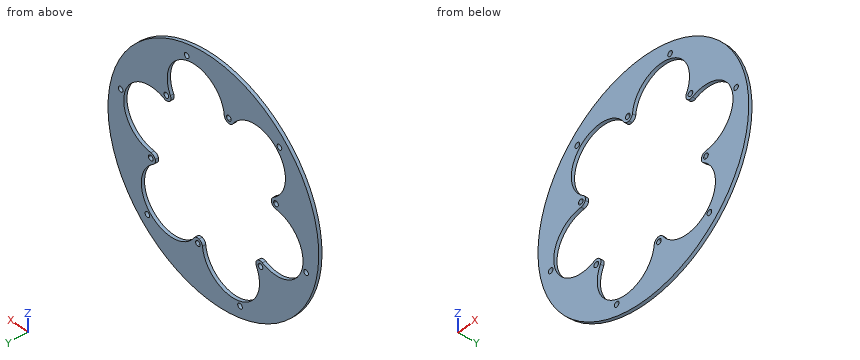
from build123d import *

# Parameters (mm, degrees)
SKETCH1_R           = 90.5
SKETCH1_R_2         = 2
BOSS_EXTRUDE1_DEPTH = 2.5


with BuildPart() as part:
    # Sketch1 → Boss-Extrude1 (new body)
    with BuildSketch(Plane(origin=(0, 0, 0), x_dir=(1, 0, 0), z_dir=(0, 1, 0))):
        with Locations(Location((0, 0, 0), (0, 0, 270))):
            Circle(SKETCH1_R)
        with Locations(Location((-56.728619257, -59.210334885, 0), (0, 0, 270))):
            Circle(SKETCH1_R_2, mode=Mode.SUBTRACT)
        with BuildLine():
            ThreePointArc((-13.809474495, -56.333511054), (-15.279862915, -53.913851845), (-12.857122546, -52.448545769))
            ThreePointArc((-12.857122546, -52.448545769), (-11.756930203, -53.155944826), (-11.329221048, -54.392027954))
            ThreePointArc((-11.329221048, -54.392027954), (-12.096441038, -55.966909996), (-13.809474495, -56.333511054))
        make_face(mode=Mode.SUBTRACT)
        with BuildLine():
            ThreePointArc((-55.690988904, -16.207399802), (-54.330696771, -13.724176472), (-51.8503343, -15.08967814))
            ThreePointArc((-51.8503343, -15.08967814), (-51.789803118, -15.36823597), (-51.769488495, -15.652569937))
            ThreePointArc((-51.769488495, -15.652569937), (-53.48931071, -17.632847798), (-55.690988904, -16.207399802))
        make_face(mode=Mode.SUBTRACT)
        with Locations(Location((22.913344548, -78.733592841, 0), (0, 0, 270))):
            Circle(SKETCH1_R_2, mode=Mode.SUBTRACT)
        with BuildLine():
            ThreePointArc((41.88151441, -40.126111252), (39.050833856, -40.189675373), (38.993211754, -37.358867629))
            ThreePointArc((38.993211754, -37.358867629), (41.183869698, -36.882833205), (42.440267447, -38.739458017))
            ThreePointArc((42.440267447, -38.739458017), (42.295327275, -39.486955868), (41.88151441, -40.126111252))
        make_face(mode=Mode.SUBTRACT)
        with Locations(Location((79.641963805, -19.523257956, 0), (0, 0, 270))):
            Circle(SKETCH1_R_2, mode=Mode.SUBTRACT)
        with Locations(Location((-79.641963805, 19.523257956, 0), (0, 0, 270))):
            Circle(SKETCH1_R_2, mode=Mode.SUBTRACT)
        with BuildLine():
            ThreePointArc((-38.993211754, 37.358867629), (-41.823892307, 37.295303508), (-41.88151441, 40.126111252))
            ThreePointArc((-41.88151441, 40.126111252), (-39.690856466, 40.602145676), (-38.434458716, 38.745520864))
            ThreePointArc((-38.434458716, 38.745520864), (-38.579398889, 37.998023012), (-38.993211754, 37.358867629))
        make_face(mode=Mode.SUBTRACT)
        with Locations(Location((-22.913344548, 78.733592841, 0), (0, 0, 270))):
            Circle(SKETCH1_R_2, mode=Mode.SUBTRACT)
        with BuildLine():
            ThreePointArc((-36.887220248, 40.576808173), (-21.946513181, 75.411419289), (9.353262234, 54.033886264))
            ThreePointArc((9.353262234, 54.033886264), (10.301978002, 51.784964754), (12.380944998, 50.506056707))
            ThreePointArc((12.380944998, 50.506056707), (14.815689048, 50.678483436), (16.696936559, 52.233673896))
            ThreePointArc((16.696936559, 52.233673896), (54.33494825, 56.711947584), (51.471349286, 18.916780429))
            ThreePointArc((51.471349286, 18.916780429), (49.998084012, 16.970707718), (49.930000652, 14.530815462))
            ThreePointArc((49.930000652, 14.530815462), (51.296698605, 12.508478628), (53.584156807, 11.656865723))
            ThreePointArc((53.584156807, 11.656865723), (76.28146143, -18.699471706), (42.118087053, -35.117105834))
            ThreePointArc((42.118087053, -35.117105834), (39.69610601, -34.814257036), (37.549055654, -35.975241245))
            ThreePointArc((37.549055654, -35.975241245), (36.481009557, -38.170004808), (36.887220248, -40.576808173))
            ThreePointArc((36.887220248, -40.576808173), (21.946513181, -75.411419289), (-9.353262234, -54.033886264))
            ThreePointArc((-9.353262234, -54.033886264), (-10.301978002, -51.784964754), (-12.380944998, -50.506056707))
            ThreePointArc((-12.380944998, -50.506056707), (-14.815689048, -50.678483436), (-16.696936559, -52.233673896))
            ThreePointArc((-16.696936559, -52.233673896), (-54.33494825, -56.711947584), (-51.471349286, -18.916780429))
            ThreePointArc((-51.471349286, -18.916780429), (-49.998084012, -16.970707718), (-49.930000652, -14.530815462))
            ThreePointArc((-49.930000652, -14.530815462), (-51.296698605, -12.508478628), (-53.584156807, -11.656865723))
            ThreePointArc((-53.584156807, -11.656865723), (-76.28146143, 18.699471706), (-42.118087053, 35.117105834))
            ThreePointArc((-42.118087053, 35.117105834), (-39.69610601, 34.814257036), (-37.549055654, 35.975241245))
            ThreePointArc((-37.549055654, 35.975241245), (-36.481009557, 38.170004808), (-36.887220248, 40.576808173))
        make_face(mode=Mode.SUBTRACT)
        with BuildLine():
            ThreePointArc((55.690988904, 16.207399802), (55.751520087, 15.928841972), (55.771834709, 15.644508005))
            ThreePointArc((55.771834709, 15.644508005), (54.052012494, 13.664230143), (51.8503343, 15.08967814))
            ThreePointArc((51.8503343, 15.08967814), (53.210626433, 17.572901469), (55.690988904, 16.207399802))
        make_face(mode=Mode.SUBTRACT)
        with BuildLine():
            ThreePointArc((13.809474495, 56.333511054), (14.909666838, 55.626111996), (15.337375993, 54.390028868))
            ThreePointArc((15.337375993, 54.390028868), (14.570156003, 52.815146826), (12.857122546, 52.448545769))
            ThreePointArc((12.857122546, 52.448545769), (11.386734126, 54.868204977), (13.809474495, 56.333511054))
        make_face(mode=Mode.SUBTRACT)
        with Locations(Location((56.728619257, 59.210334885, 0), (0, 0, 270))):
            Circle(SKETCH1_R_2, mode=Mode.SUBTRACT)
    extrude(amount=BOSS_EXTRUDE1_DEPTH)


solid = part.part
Verification items for the finished model (mm, model axes). Coordinates: 2 decimals unless noted, no trailing zeros. Order: outer loops, then holes, each group sorted by start corner. A loop starts at its lowest first (then second) coordinate and runs counter-clockwise, first axis right, second up. Notation, with made-up numbers: M -6.5,68 L 33.5,68 A27 cw 33.5,84 Z; hole C 61.5,57 d8. An arc over 180 degrees is marked long. One line per item, written item: value. Start each with the question number.
Item 1: Sectioned sample at C-C on y = 1.55. Give the number of separate pieces and of enclosed holes in the cut face, then the cut area to 3 significant figures.
Item 2: Sectioned sample at B-B on x = 0. Record the cut outline in (y, z), then the cut area to 3 significant figures.
Item 3: Thickness scan on probe 1 along X at (y, z) = (1.7, -58.5); probe 2 along Z at (x, y) = (-37, 0.55); probe 3 along X at (y, z) = (2.2, -59). Record the ranges inside material, lowest first.
Item 4: Sectioned sample at A-A on z = 32. Record the cut outline in (x, y).
Calculated:
1. separate pieces: 1
1. enclosed holes: 13
1. area: 10,200 mm^2
2. outline: M 0,-90.5 L 2.5,-90.5 L 2.5,-71.2 L 0,-71.2 Z; M 0,71.2 L 2.5,71.2 L 2.5,90.5 L 0,90.5 Z
2. area: 96.5 mm^2
3. probe 1: -69.05 to -38.71, 8.53 to 22.47, 52.25 to 54.86, 58.6 to 69.05
3. probe 2: -82.59 to -62.9, -40.8 to -36.7, 63.53 to 82.59
3. probe 3: -68.62 to -38.56, 8.39 to 23.15, 51.57 to 54.74, 58.72 to 68.62
4. outline: M -84.65,0 L -60.88,0 L -60.88,2.5 L -84.65,2.5 Z; M 67.8,0 L 84.65,0 L 84.65,2.5 L 67.8,2.5 Z
